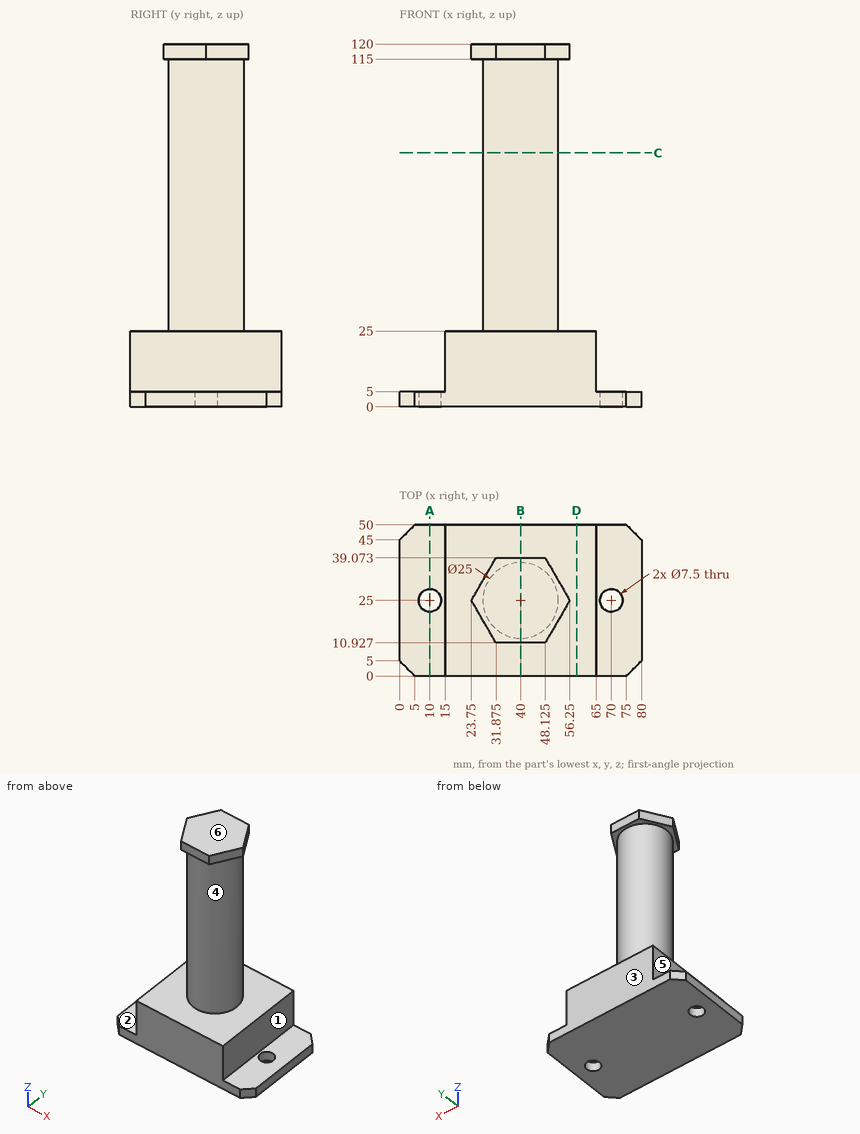
Study the drawing (mm; zero at the part's minimum x, y, z) and answer. A direction names the side the tool comes from. Round coordinates to 2 decimals unless told otherwise and drop trailing zeros. Loops run counter-clockwise (first coordinate to the right, second up) from the corner with the lowest first, then second, coordinate; pieces in that order, holes last. Notation, with made-up numbers: (85.5, 87) -> (104.5, 87) arc R21 ccw to (104.5, 117) -> close; hole circle Ø5 at (88.25, 56.5). An arc over 180 degrees is marked (long way). Write each question's results on one line, items separated by ' | '. Start each with the question number.
1. Given pin 1 Ø1.5 at (x, z) = (38, 118.5) entering from +Y; pin 2 Ø6 at (x, y) = (16.5, 26) entering from +Z; pin 3 Ø4.5 at (x, y) = (10.5, 18.5) entering from +Z, each flat-ended and moving along its own axis, determine where each tip first touches the part or whether it passes through.
2. Section C-C (z = 84) is taken. Determine the outline of the cut face in (x, y), plus the area to 3 significant figures.
3. Section D-D (x = 58.5) is taken. Determine the outline of the cut face in (y, z), plus the area to 3 significant figures.
4. Find the intervals of material crossed by probe 1 along X at (y, z) = (25, 3.65); probe 2 along Y at (x, z) = (70, 1.05); probe 3 along Z at (x, y) = (19, 29), in increasing order. Write a range as from..to.
5. Section B-B (x = 40) is taken. Determine the outline of the cut face in (y, z), plus the area to 3 significant figures.
6. Section A-A (x = 10) is taken. Determine the outline of the cut face in (y, z), plus the area to 4 significant figures.
7. For a pull along Z with two mould halves and no side action, classify the marked faces 4, 5 and 6 as +Z half, -Z half, draft (parallel to the pull), parting line (faces both ways), or undercut.
8. A tool of negligible diameter and unlimited length cuts with its end or side. For the marked faces 1, 2 and 3, from which of +Z, -Z, +X, -X, +Y, -Y can it reach the whole face along a straight path? Write none if from no direction.
Evaluation:
1) pin 1: stops at y = 39.07 | pin 2: stops at z = 25 | pin 3: stops at z = 5
2) outline: circle Ø25 at (40, 25) | area: 491 mm2
3) outline: (0, 0) -> (50, 0) -> (50, 25) -> (0, 25) -> close | area: 1,250 mm2
4) probe 1: x = 0..6.25, 13.75..66.25, 73.75..80 | probe 2: y = 0..21.25, 28.75..50 | probe 3: z = 0..25
5) outline: (0, 0) -> (50, 0) -> (50, 25) -> (37.5, 25) -> (37.5, 115) -> (39.07, 115) -> (39.07, 120) -> (10.93, 120) -> (10.93, 115) -> (12.5, 115) -> (12.5, 25) -> (0, 25) -> close | area: 3,640 mm2
6) outline: (0, 0) -> (21.25, 0) -> (21.25, 5) -> (0, 5) -> close; (28.75, 0) -> (50, 0) -> (50, 5) -> (28.75, 5) -> close | area: 212.5 mm2
7) face 4: undercut | face 5: draft | face 6: +Z half
8) face 1: +Z, +X, +Y, -Y | face 2: +Z, -X, +Y, -Y | face 3: +Z, -Z, +X, -X, +Y
